The model under review builds one solid part; all positions refer to its coordinate system, in mm. Coordinates: 2 decimals unless noted, no trailing zeros. Write each loop counter-clockwise with the first axis right and the second up, starting at its lowest first coordinate (ties: lowest second). Pieces come first, ordered by that corner, then holes. Notation, with made-up numbers: (0, 49) - (17, 49) arc R7 cw to (17, 53) - close; hole circle Ø1 at (23.25, 84.5). An arc over 180 degrees is marked (long way). Return JSON: item names as keys, results as strings. Group by question number.
(1) To check wall thickness, follow L1, parallel to X at y = -1, z = 1.25; L2, parallel to X at y = 13.5, z = 3.25; L3, parallel to X at y = 28, z = 0.6. State the ranges of each line that lie inside material, in increasing order. Write a range as from..to.
(2) For pin 1 Ø1 at (y, z) = (4, 3) entering from +X; pin 2 Ø2 at (x, z) = (-4, 0.5) entering from -Y; pin 3 Ø2 at (x, z) = (1.5, 1.5) entering from -Y, all flat-tipped, find the tip position at first contact; note any pin that passes through.
(3) We need section D-D on y = -18. State the section outline as (x, z) points.
(4) We need section B-B on y = 0. State the section outline as (x, z) points.
(5) We need section C-C on z = 2.9. State the section outline as (x, y) points.
(6) We need section A-A on x = 0. State the section outline as (y, z) points.
(7) Draft analysis for pull direction X (two halves, no side actions). For faces 1 (the face through (30.76, 9.69, 1.97)), 2 (the face through (-0.767, -39.993, 1.972)), 3 (the face through (-43.766, 6.316, 1.972)), state which applies: released by +X, released by -X, zero draft, split by the parting line, or undercut.
```python
from build123d import *

# Parameters (mm, degrees)
SKETCH_1_R      = 40
SKETCH_1_R_2    = 32.25
EXTRUDE_1_DEPTH = 4
SKETCH_2_R      = 1.6
EXTRUDE_2_DEPTH = 4


with BuildPart() as part:
    # 草图1 → 凸台-拉伸1 (new body)
    with BuildSketch(Plane.XY):
        Circle(SKETCH_1_R)
        Circle(SKETCH_1_R_2, mode=Mode.SUBTRACT)
    extrude(amount=EXTRUDE_1_DEPTH)

    # 草图2 → 凸台-拉伸2 (add)
    # profile 1 of 2: a face of its own
    with BuildSketch(Plane(origin=(0, 0, 0), x_dir=(-1, 0, 0), z_dir=(0, 0, -1))):
        with BuildLine():
            Line((48.210100717, 4.698463104), (39.196053971, 7.97930781))
            ThreePointArc((39.196053971, 7.97930781), (40, 0), (39.196053971, -7.97930781))
            Line((39.196053971, -7.97930781), (48.210100717, -4.698463104))
            ThreePointArc((48.210100717, -4.698463104), (51.5, 0), (48.210100717, 4.698463104))
        make_face()
        with Locations((46.5, 0)):
            Circle(SKETCH_2_R, mode=Mode.SUBTRACT)
    # profile 2 of 2: a face of its own
    with BuildSketch(Plane(origin=(0, 0, 0), x_dir=(-1, 0, 0), z_dir=(0, 0, -1))):
        with BuildLine():
            Line((-48.210100717, -4.698463104), (-39.196053971, -7.97930781))
            ThreePointArc((-39.196053971, -7.97930781), (-40, 0), (-39.196053971, 7.97930781))
            Line((-39.196053971, 7.97930781), (-48.210100717, 4.698463104))
            ThreePointArc((-48.210100717, 4.698463104), (-51.5, 0), (-48.210100717, -4.698463104))
        make_face()
        with Locations(Location((-46.5, 0, 0), (0, 0, 180))):
            Circle(SKETCH_2_R, mode=Mode.SUBTRACT)
    extrude(amount=-EXTRUDE_2_DEPTH)


solid = part.part
```
Ans:
{
 "1": {"L1": "-51.4..-47.75, -45.25..-32.23, 32.23..45.25, 47.75..51.4", "L2": "-37.65..-29.29, 29.29..37.65", "L3": "-28.57..-16, 16..28.57"},
 "2": {"pin 1": "x = 50.07", "pin 2": "y = -39.89", "pin 3": "y = -40"},
 "3": {"outline": "(-35.72, 0) - (-26.76, 0) - (-26.76, 4) - (-35.72, 4) - close; (26.76, 0) - (35.72, 0) - (35.72, 4) - (26.76, 4) - close"},
 "4": {"outline": "(-51.5, 0) - (-48.1, 0) - (-48.1, 4) - (-51.5, 4) - close; (-44.9, 0) - (-32.25, 0) - (-32.25, 4) - (-44.9, 4) - close; (32.25, 0) - (44.9, 0) - (44.9, 4) - (32.25, 4) - close; (48.1, 0) - (51.5, 0) - (51.5, 4) - (48.1, 4) - close"},
 "5": {"outline": "(-48.21, -4.7) - (-39.2, -7.98) arc R40 ccw to (39.2, -7.98) - (48.21, -4.7) arc R5 ccw to (48.21, 4.7) - (39.2, 7.98) arc R40 ccw to (-39.2, 7.98) - (-48.21, 4.7) arc R5 ccw to start; hole circle Ø3.2 at (-46.5, 0); hole circle Ø64.5 at (0, 0); hole circle Ø3.2 at (46.5, 0)"},
 "6": {"outline": "(-40, 0) - (-32.25, 0) - (-32.25, 4) - (-40, 4) - close; (32.25, 0) - (40, 0) - (40, 4) - (32.25, 4) - close"},
 "7": {"face 1": "undercut", "face 2": "split by the parting line", "face 3": "released by -X"}
}
